Can you work these out from the model? Positions are in its coordinate system, mm. A direction names the side the tool comes from. Round coordinates to 2 decimals unless told otherwise and drop trailing zeros. Loops run counter-clockwise (first coordinate to the right, second up) from the corner with the lowest first, then second, coordinate; pieces in that order, holes last. Notation, with made-up numbers: M -24.5,-31.75 L 23.5,-31.75 A27 ccw 23.5,-10.75 Z; hole C 57.25,57 d3. An arc over 180 degrees is marked long. Answer as CSV lines item,"result".
from build123d import *

# Parameters (mm, degrees)
F0_W     = 7
F0_H     = 10
F1_DEPTH = 6
F0_W_2   = 186
F2_DEPTH = 0.4


with BuildPart() as f1:
    # F0 (on Top) → F1 (new body)
    with BuildSketch(Plane.XY):
        with Locations((-96.5, -5)):
            Rectangle(F0_W, F0_H)
    extrude(amount=-F1_DEPTH)



with BuildPart() as f1b:
    # F0 (on Top) → F1, piece 2 (new body)
    with BuildSketch(Plane.XY):
        with Locations((96.5, -5)):
            Rectangle(F0_W, F0_H)
    extrude(amount=-F1_DEPTH)


with BuildPart() as f1_1:
    add(f1.part)

    add(f1b.part)  # F2 merges F1b
    # F0 (on Top) → F2 (join)
    with BuildSketch(Plane.XY):
        with Locations((-96.5, -5)):
            Rectangle(F0_W, F0_H)
        with Locations((0, -5)):
            Rectangle(F0_W_2, F0_H)
        with Locations((96.5, -5)):
            Rectangle(F0_W, F0_H)
    extrude(amount=F2_DEPTH)


solid = f1_1.part
Item 1: On a 3-axis mill with a long thin cutter (end or side, diameter ignored), from which of +Z, -Z, +X, -X, +Y, -Y can I reach the whole of each face in a straight line? I mean faces 1 (the face through (-93, -5, -3)), 2 (the face through (96, -5, -6)). Say none if no direction works.
Output:
face 1,"-Z, +Y, -Y"
face 2,"-Z, +X, -X, +Y, -Y"
Item 2: Will this pin go through, and if not, where does the flat tip stop? pin 1 (1 mm diameter, centred on x = 5, y = -6, fed in from -Z).
Output:
pin 1,"stops at z = 0"
Item 3: If I drill on line 1 along X through (y, z) = (-5.5, -0.25); line 2 along Z through (x, y) = (41, -2.5), over which ranges is the centre line in solid material (lowest first)? Write a range as from..to.
Output:
line 1,"x = -100..-93, 93..100"
line 2,"z = 0..0.4"
Item 4: If we section it at A-A on z = -1.75: Write out the boundary of the cut face in (x, y), then the cut area to 3 significant figures.
Output:
outline,"M -100,-10 L -93,-10 L -93,0 L -100,0 Z; M 93,-10 L 100,-10 L 100,0 L 93,0 Z"
area,"140 mm2"
Item 5: If we section it at C-C on x = -85.5: Write out the boundary of the cut face in (y, z).
Output:
outline,"M -10,0 L 0,0 L 0,0.4 L -10,0.4 Z"
Item 6: If we section it at B-B on y = -5.5: Write out the boundary of the cut face in (x, z).
Output:
outline,"M -100,-6 L -93,-6 L -93,0 L 93,0 L 93,-6 L 100,-6 L 100,0.4 L -100,0.4 Z"
